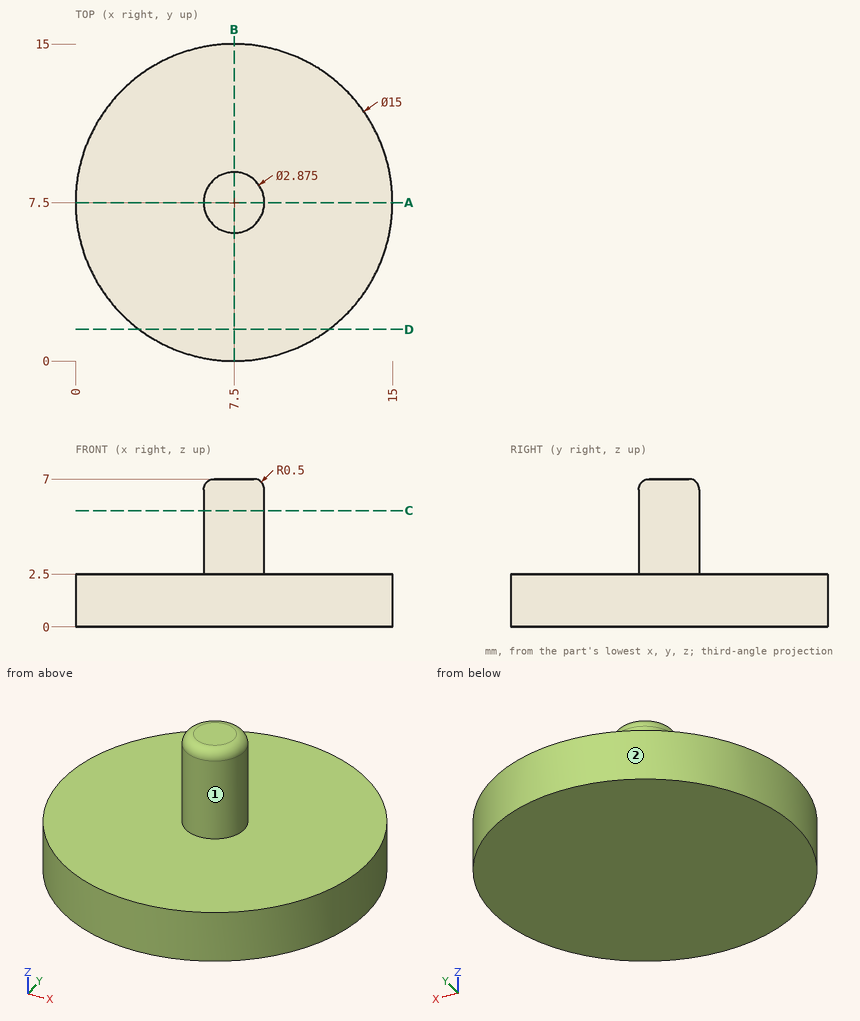
Verification items for this drawing (mm, ordinates from the low corner). A direction names the side the tool comes from. Give positions to 0.01 mm unless a question says otherwise; leave off trailing zeros. Write each loop counter-clockwise with the first axis right and the second up, starting at its lowest first coordinate (ties: lowest second). Pieces come first, ordered by that corner, then holes.
1) Cross-section at A-A (y = 7.5). Record the boundary of the cut face in (x, z), plus the area to 3 significant figures.
Values follow:
outline: (0, 0) - (15, 0) - (15, 2.5) - (8.94, 2.5) - (8.94, 6.5) arc R0.5 ccw to (8.44, 7) - (6.56, 7) arc R0.5 ccw to (6.06, 6.5) - (6.06, 2.5) - (0, 2.5) - close
area: 50.3 mm2
2) Cross-section at C-C (z = 5.5). Record the boundary of the cut face in (x, y) (1 decimal), plus the area to 3 significant figures.
Values follow:
outline: circle Ø2.9 at (7.5, 7.5)
area: 6.49 mm2
3) Cross-section at D-D (y = 1.5). Record the boundary of the cut face in (x, z), plus the area to 3 significant figures.
Values follow:
outline: (3, 0) - (12, 0) - (12, 2.5) - (3, 2.5) - close
area: 22.5 mm2
4) Go/stop test with flat-tipped pins: pin 1 Ø6 at (x, y) = (3.5, 5) entering from +Z; pin 2 Ø1.5 at (x, z) = (3.5, 1.5) entering from +Y; pin 3 Ø4 at (y, z) = (12.5, 1.5) entering from -X. Record where each tip stops, or that it passes through.
Values follow:
pin 1: stops at z = 2.5
pin 2: stops at y = 14.26
pin 3: stops at x = 0.63
5) Set-up check for the marked faces 1 and 2: record each of +Z, -Z, +X, -X, +Y, -Y from which the full face is reachable in a straight line by a thin tool's end or side.
Values follow:
face 1: +Z
face 2: +Z, -Z
6) Thickness scan on line 1 (Z direction, x = 13, y = 4.5); line 2 (Y direction, x = 3.75, z = 1.75); line 3 (Y direction, x = 10.25, z = 1.75). Record the ranges inside material, lowest first.
Values follow:
line 1: z = 0 to 2.5
line 2: y = 1 to 14
line 3: y = 0.52 to 14.48
